Read the model definition and answer for the solid it produces. Units are mm, in the model's axes. A direction names the side the tool comes from. Round coordinates to 2 decimals unless told otherwise and drop trailing zeros. Write each loop counter-clockwise with the first axis right and the second up, starting at its lowest first coordinate (ties: lowest second). Pieces come first, ordered by that corner, then holes. Notation, with made-up numbers: (76, -36.75) - (133, -36.75) arc R19 cw to (133, -22.75) - close; hole circle Ø10 at (56, -21.5). An arc over 180 degrees is marked (long way). Answer as CSV lines item,"result". Start each with the question number.
1) Find section A-A on y = 68.5. Determine the outline of the cut face in (x, z), then the cut area to 3 significant figures.
2) Each of these flat-tipped pins is pushed along its axis until it touches: pin 1 (8 mm diameter, centred on x = 1.5, y = 138, fed in from -Z); pin 2 (1 mm diameter, centred on y = 135, z = 0, fed in from -X); pin 3 (5 mm diameter, centred on x = 8, y = 48, fed in from -Z). Where does it stop, or does it pass through?
3) Find section B-B on y = 35. Determine the outline of the cut face in (x, z).
4) Which of the six approach directions +Z, -Z, +X, -X, +Y, -Y give full straight-line access (tool end or side, diameter ignored) to faces 1 (the conical face through (6.012, 83.456, 1.893)), 2 (the cylindrical face through (-1.22, 3.13, -9.32))?
5) Consider line 1 along Z through (x, y) = (3.25, 58); line 2 along X through (y, z) = (128, 1.25); line 3 along Z through (x, y) = (-6.75, 66). Determine where each line is inside the solid, lowest interval first.
from build123d import *

# Parameters (mm, degrees)
SKETCH1_R           = 9.398
BOSS_EXTRUDE1_DEPTH = 6.35
FILLET1_R           = 0.889


with BuildPart() as part:
    # Sketch1 → Boss-Extrude1 (new body)
    with BuildSketch(Plane(origin=(0, 0, 0), x_dir=(1, 0, 0), z_dir=(0, 1, 0))):
        Circle(SKETCH1_R)
    extrude(amount=BOSS_EXTRUDE1_DEPTH)

    # Sketch2 → Revolve1 (revolve)
    with BuildSketch(Plane.XY):
        Polygon((11.811, 6.35), (0.889, 159.258), (0, 159.258), (0, 6.35), align=None)
    revolve(axis=Axis((0, 159.258, 0), (0, -1, 0)))

    # Fillet1
    fillet1_edges = [part.edges().sort_by_distance(p)[0] for p in [
        (-0.889, 159.258, 0),
    ]]
    fillet(fillet1_edges, radius=FILLET1_R)


solid = part.part
Check values:
1,outline,"circle Ø14.74 at (0, 0)"
1,area,"171 mm^2"
2,pin 1,"stops at z = -2.67"
2,pin 2,"stops at x = -2.66"
2,pin 3,"stops at z = -6.93"
3,outline,"circle Ø19.53 at (0, 0)"
4,face 1,"+Y"
4,face 2,"-Y"
5,line 1,"z = -7.44 to 7.44"
5,line 2,"x = -2.86 to 2.86"
5,line 3,"z = -3.38 to 3.38"
